The model under review builds one solid part; all positions refer to its coordinate system, in mm. A direction names the side the tool comes from. Round coordinates to 2 decimals unless told otherwise and drop trailing zeros. Loops run counter-clockwise (first coordinate to the right, second up) from the corner with the lowest first, then second, coordinate; pieces in that order, holes last. Notation, with made-up numbers: (-26.5, -23.75) -> (-10.5, -23.75) arc R20 ccw to (-10.5, -11.75) -> close; hole circle Ø2 at (43.5, -14). An arc over 180 degrees is marked (long way). Use a Markdown table: item, result. Add a question column.
1) Consider section B-B on x = 0. Give the boundary of the cut face in (y, z).
2) Insertion check: pin 1 (2 mm diameter, centred on x = -13, y = -10, fed in from +Z); pin 2 (1 mm diameter, centred on x = 9.5, y = -6, fed in from +Z); pin 3 (5 mm diameter, centred on x = -14.5, z = 3.5, fed in from +Y); pin 4 (12 mm diameter, centred on y = -6, z = -12, fed in from -X). Each pin has a flat end and moves straight along its axis. Give the tip position at first contact, or say it passes through.
3) Consider section C-C on y = -11. Give the boundary of the cut face in (x, z).
4) For faces 1 (the cylindrical face through (-16.8, -25.5, 5.1)), 2 (the cylindrical face through (17.169, -19.841, 5.407)), list the 3-axis set-ups (+Z, -Z, +X, -X, +Y, -Y) from which the entire face can be reached by the end or side of a thin tool; tool diameter is ignored.
5) Mouldability with a two-part tool opening along Y and no side actions: class faces 3 (the cylindrical face through (-11.05, -21.08, -4.88)), 4 (the conical face through (-2.886, -0.542, -12.996)), 5 (the conical face through (-2.886, -39.458, -12.996)) as released by +Y, released by -Y, zero draft, split by the parting line, or undercut.
6) Consider section A-A on z = 0. Give the boundary of the cut face in (x, y), plus the area to 3 significant figures.
7) Consider section D-D on y = -20. Give the boundary of the cut face in (x, z) (3 decimals).
8) Wall thickness on probe 1 along Z at (x, y) = (0, -14); probe 2 along Z at (x, y) = (-13.75, -20); probe 3 along X at (y, z) = (-24, -5.5): over which ranges is each line inside the solid? List them lowest first.
from build123d import *

# Parameters (mm, degrees)
F0_R     = 18
F0_R_2   = 8
F1_DEPTH = 40
F2_R     = 5
F3_DEPTH = 25
F5_R     = 7.5
F6_DEPTH = 2
F7_SIZE  = 1
F8_SIZE2 = 8.660254
F8_SIZE  = 5


with BuildPart() as f1:
    # F0 (on Front) → F1 (new body)
    with BuildSketch(Plane.XZ):
        Circle(F0_R)
        Circle(F0_R_2, mode=Mode.SUBTRACT)
    extrude(amount=F1_DEPTH)

    # F2 (on Right) → F3 (cut)
    with BuildSketch(Plane.YZ):
        with Locations((-20, 0)):
            Circle(F2_R)
    extrude(amount=-F3_DEPTH, mode=Mode.SUBTRACT)

    # F5 (on offset) → F6 (cut)
    with BuildSketch(Plane.YZ.offset(-18)):
        with Locations((-20, 0)):
            Circle(F5_R)
    extrude(amount=F6_DEPTH, mode=Mode.SUBTRACT)

    # F7
    f7_edges = [f1.edges().sort_by_distance(p)[0] for p in [
        (-8, -40, 0),
        (-8, 0, 0),
    ]]
    chamfer(f7_edges, length=F7_SIZE)

    # F8
    f8_edges = [f1.edges().sort_by_distance(p)[0] for p in [
        (-18, -40, 0),
        (-18, 0, 0),
    ]]
    chamfer(f8_edges, length=F8_SIZE, length2=F8_SIZE2)


solid = f1.part
Result set:
| question | item | result |
|---|---|---|
| 1 | outline | (-40, -13) -> (-31.34, -18) -> (-8.66, -18) -> (0, -13) -> (0, -9) -> (-1, -8) -> (-39, -8) -> (-40, -9) -> close; (-40, 9) -> (-39, 8) -> (-1, 8) -> (0, 9) -> (0, 13) -> (-8.66, 18) -> (-31.34, 18) -> (-40, 13) -> close |
| 2 | pin 1 | z = 13.42 |
| 2 | pin 2 | z = 13.93 |
| 2 | pin 3 | y = 0 |
| 2 | pin 4 | x = -16.74 |
| 3 | outline | circle Ø36 at (0, 0); hole circle Ø16 at (0, 0) |
| 4 | face 1 | -X |
| 4 | face 2 | +Y, -Y |
| 5 | face 3 | undercut |
| 5 | face 4 | released by +Y |
| 5 | face 5 | released by -Y |
| 6 | outline | (-18, -31.34) -> (-13, -40) -> (-9, -40) -> (-8, -39) -> (-8, -25) -> (-16, -25) -> (-16, -27.5) -> (-18, -27.5) -> close; (-18, -12.5) -> (-16, -12.5) -> (-16, -15) -> (-8, -15) -> (-8, -1) -> (-9, 0) -> (-13, 0) -> (-18, -8.66) -> close; (8, -39) -> (9, -40) -> (13, -40) -> (18, -31.34) -> (18, -8.66) -> (13, 0) -> (9, 0) -> (8, -1) -> close |
| 6 | area | 601 mm2 |
| 7 | outline | (-16.363, -7.5) arc R18 ccw (long way) to (-16.363, 7.5) -> (-16, 7.5) -> (-16, 5) -> (-6.245, 5) arc R8 cw (long way) to (-6.245, -5) -> (-16, -5) -> (-16, -7.5) -> close |
| 8 | probe 1 | -18 to -8, 8 to 18 |
| 8 | probe 2 | -11.62 to -5, 5 to 11.62 |
| 8 | probe 3 | -16 to -5.81, 5.81 to 17.14 |
